Can you work these out from the model? Positions are in its coordinate system, mm. Face numbers are marked on the shaded views. A direction names the side the tool comes from. Give positions to 0.01 mm unless a question says otherwise; leave off trailing zeros. Write each loop counter-clockwise with the first axis right and the second up, starting at its lowest first coordinate (ties: lowest second). Pieces come first, ordered by that corner, then holes.
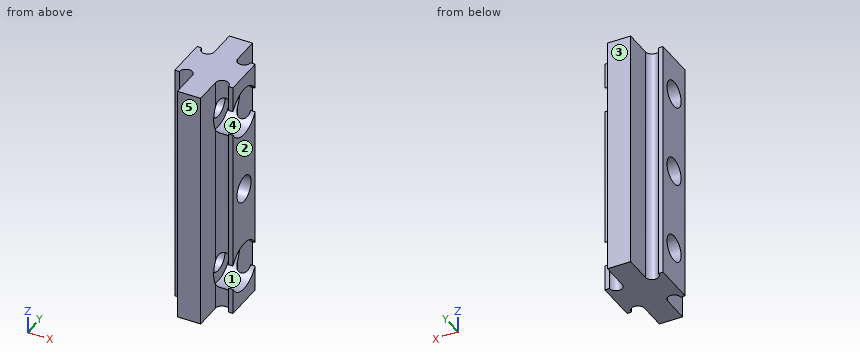
from build123d import *

# Parameters (mm, degrees)
BOSS_EXTRUDE1_DEPTH = 23.8125
SKETCH2_R           = 2.5796875
CUT_EXTRUDE1_DEPTH  = 12.43
SKETCH3_R           = 4.7625
CUT_EXTRUDE2_DEPTH  = 5.08


with BuildPart() as part:
    # Sketch1 → Boss-Extrude1 (new body, symmetric)
    with BuildSketch(Plane.XY):
        with BuildLine():
            Line((0, -9.525), (0, 9.525))
            Line((0, 9.525), (-2.286, 9.525))
            Line((-2.286, 9.525), (-2.286, 4.064))
            ThreePointArc((-2.286, 4.064), (-3.556, 2.794), (-4.826, 4.064))
            Line((-4.826, 4.064), (-5.715, 4.064))
            Line((-5.715, 4.064), (-5.715, -4.064))
            Line((-5.715, -4.064), (-4.826, -4.064))
            ThreePointArc((-4.826, -4.064), (-3.556, -2.794), (-2.286, -4.064))
            Line((-2.286, -4.064), (-2.286, -9.525))
            Line((-2.286, -9.525), (0, -9.525))
        make_face()
    boss_extrude1 = extrude(amount=BOSS_EXTRUDE1_DEPTH, both=True)

    # Mirror1: Boss-Extrude1 across plane
    add(boss_extrude1.mirror(Plane(origin=(0, -9.525, 23.8125), x_dir=(0, 0, 1), z_dir=(-1, 0, 0))))

    # Sketch2 → Cut-Extrude1 (cut, through all)
    with BuildSketch(Plane(origin=(5.715, 0, 0), x_dir=(0, 0, -1), z_dir=(1, 0, 0))):
        with Locations((-16.2814, 0)):
            Circle(SKETCH2_R)
        with Locations((16.2814, 0)):
            Circle(SKETCH2_R)
        Circle(SKETCH2_R)
    extrude(amount=-CUT_EXTRUDE1_DEPTH, mode=Mode.SUBTRACT)

    # Sketch3 → Cut-Extrude2 (cut)
    with BuildSketch(Plane(origin=(5.715, 0, 0), x_dir=(0, 0, -1), z_dir=(1, 0, 0))):
        with Locations((-16.2814, 0)):
            Circle(SKETCH3_R)
        with Locations((16.2814, 0)):
            Circle(SKETCH3_R)
    extrude(amount=-CUT_EXTRUDE2_DEPTH, mode=Mode.SUBTRACT)


solid = part.part
(1) Imagine slicing it at C-C, the plane z = 0. Write out the boundary of the cut face in (x, y) (3 decimals).
Returned:
outline: (-5.715, -4.064) - (-4.826, -4.064) arc R1.27 cw to (-2.286, -4.064) - (-2.286, -9.525) - (2.286, -9.525) - (2.286, -4.064) arc R1.27 cw to (4.826, -4.064) - (5.715, -4.064) - (5.715, -2.58) - (-5.715, -2.58) - close; (-5.715, 2.58) - (5.715, 2.58) - (5.715, 4.064) - (4.826, 4.064) arc R1.27 cw to (2.286, 4.064) - (2.286, 9.525) - (-2.286, 9.525) - (-2.286, 4.064) arc R1.27 cw to (-4.826, 4.064) - (-5.715, 4.064) - close
(2) Imagine slicing it at B-B, the plane x = 3.5. Write out the boundary of the cut face in (y, z) (1 decimal).
Returned:
outline: (-2.8, -23.8) - (2.8, -23.8) - (2.8, -20.1) arc R4.8 cw to (-2.8, -20.1) - close; (-2.8, -12.4) arc R4.8 cw to (2.8, -12.4) - (2.8, 12.4) arc R4.8 cw to (-2.8, 12.4) - close; (-2.8, 20.1) arc R4.8 cw to (2.8, 20.1) - (2.8, 23.8) - (-2.8, 23.8) - close; hole circle Ø5.2 at (0, 0)
(3) Imagine slicing it at A-A, the plane y = 0. Write out the boundary of the cut face in (x, z) (1 decimal).
Returned:
outline: (-5.7, -23.8) - (5.7, -23.8) - (5.7, -21) - (0.6, -21) - (0.6, -18.9) - (-5.7, -18.9) - close; (-5.7, -13.7) - (0.6, -13.7) - (0.6, -11.5) - (5.7, -11.5) - (5.7, -2.6) - (-5.7, -2.6) - close; (-5.7, 2.6) - (5.7, 2.6) - (5.7, 11.5) - (0.6, 11.5) - (0.6, 13.7) - (-5.7, 13.7) - close; (-5.7, 18.9) - (0.6, 18.9) - (0.6, 21) - (5.7, 21) - (5.7, 23.8) - (-5.7, 23.8) - close
(4) Will these pins go through, and if not, where does the flat tip stop? P1, Ø6.5, axis at y = 0, z = 16.28, coming from the +X side (3 decimals); P2, Ø1, axis at x = -5.5, z = 5.5, coming from the +Y side; P3, Ø1, axis at x = 5, z = -5.5, coming from the -Y side.
Returned:
P1: stops at x = 0.635
P2: stops at y = 4.06
P3: stops at y = -4.06
(5) Imagine slicing it at D-D, the plane x = -1. Write out the boundary of the cut face in (y, z) (1 decimal).
Returned:
outline: (-9.5, -23.8) - (9.5, -23.8) - (9.5, 23.8) - (-9.5, 23.8) - close; hole circle Ø5.2 at (0, -16.3); hole circle Ø5.2 at (0, 0); hole circle Ø5.2 at (0, 16.3)
(6) For the marked faces 1 and 2, which set-ups out of +Z, -Z, +X, -X, +Y, -Y let a thin tool reach every point of the face, with its end or its side?
Returned:
face 1: +X
face 2: +Z, -Z, +X, +Y, -Y
(7) If we mould it in two halves opening along Y, with no side actions, what happens to the marked faces 3, 4 and 5? For each: +Y half, -Y half, draft (parallel to the pull), parting line (faces both ways), or undercut.
Returned:
face 3: +Y half
face 4: undercut
face 5: -Y half
(8) If I drill on L1, parallel to X at y = -6, z = -14.5; L2, parallel to Y at x = -3.5, z = -17.5; L3, parallel to Y at x = -1, z = -1.5 (3 decimals), over which ranges is the centre line in solid material (lowest first)?
Returned:
L1: x = -2.29 to 2.29
L2: y = -2.8 to -2.27, 2.27 to 2.8
L3: y = -9.525 to -2.099, 2.099 to 9.525
